Source: CAD feature listing. Evaluate the final solid. Frame: model axes, mm. A direction names the side the tool comes from. Coordinates: 2 decimals unless noted, no trailing zeros. Write each loop counter-clockwise with the first axis right and the second up, starting at its lowest first coordinate (ties: lowest second). Pieces come first, ordered by that corner, then holes. Notation, with made-up numbers: M -36,-25 L -23,-25 A17 cw -23,-3 Z; hole C 45,-35 d7. An arc over 180 degrees is marked long. Write item = value, one per line. Start each with the question number.
1. Pull-direction query (Y, two-part tool) for faces 1 (the face through (-8.287, -4.696, 4.16)), 2 (the face through (8.287, 4.696, 4.16)), 3 (the face through (-0.2, 6.5, 0)); classes: pulls with the +Y half, pulls with the -Y half, needs draft (parallel to the pull), parting line crosses it, or undercut.
2. Line query: line 1 along X through (y, z) = (-8, 0.5); line 2 along Z through (x, y) = (3.75, 6); line 3 along X through (y, z) = (-4, -73.5). Output: solid intervals per line, ascending.
3. Pin query (flat end, axial travel): pin 1 Ø2 at (y, z) = (-4.5, -97.5) entering from -X; pin 2 Ø4 at (x, z) = (-1.5, -141.5) entering from +Y; pin 3 Ø1 at (x, z) = (-2, -147) entering from -Y. Return the tip coordinate at first contact, or that it passes through.
4. Section query B-B (z = -158). Output: boundary loops of the cut face in (x, y), then the cut area to 3 significant figures.
5. Access query for faces 4 (the face through (6.056, -1.907, -96.163)), 5 (the face through (0, -9.525, 4)). Directions: +Z, -Z, +X, -X, +Y, -Y. A direction counts if a zero-diameter tool reaches every point of the face in a straight line with its end or side. Return the directions, or none.
Solid Edge part; units mm, degrees
sketch "Sketch1" plane through (0, 0, 0) normal (0, 0, 1) x (1, 0, 0)
  circle A0 centre (0, 0) radius 11.049
extrude "Protrusion1" add sketch "Sketch1" along normal blind 8.2042
sketch "Sketch2" plane through (0, 0, 0) normal (0, 0, -1) x (1, 0, 0)
  circle A0 centre (0, 0) radius 6.35
extrude "Protrusion2" add sketch "Sketch2" along normal blind 190.5
sketch "Sketch3" plane through (0, 0, -190.5) normal (0, 0, -1) x (1, 0, 0)
  circle A0 centre (0, 0) radius 6.3497
extrude "Cutout1" cut sketch "Sketch3" against normal blind 190.373 flip side to cut
chamfer "Chamfer_1" distance 0.9525 angle 45 1 edges at (-6.3497, 0, -190.5)
sketch "Sketch4" plane through (0, 0, 8.2042) normal (0, 0, 1) x (1, 0, 0)
  line L0 (-5.5995, 9.525) -> (5.5995, 9.525)
extrude "Cutout2" cut sketch "Sketch4" against normal up to next material side at (0, 9.575, 8.2042)
pattern_circular "Pattern1" count 6 over 360 about axis through (0, 0, 8.2042) along (0, 0, 1) of "Cutout2"
properties part number "108070"
Results are:
q1.face_1 = pulls with the -Y half
q1.face_2 = pulls with the +Y half
q1.face_3 = needs draft
q2.line_1 = -6.38 to 6.38
q2.line_2 = 0 to 8.2
q2.line_3 = -4.93 to 4.93
q3.pin_1 = -5.3
q3.pin_2 = 6.35
q3.pin_3 = -6.17
q4.outline = C 0,0 d12.7
q4.area = 127 mm^2
q5.face_4 = -Z
q5.face_5 = +Z, -Z, +X, -X, -Y
